Read the model definition and answer for the solid it produces. Units are mm, in the model's axes. Coordinates: 2 decimals unless noted, no trailing zeros.
Q1. Straight lines are drawn through the part: line 1 (Z direction, x = 117, y = -3.75); line 2 (Z direction, x = 168, y = -3.2); line 3 (X direction, y = -2.9, z = -32). For each, find the intervals that lie inside material, in ascending order.
Q2. Section A-A (x = 135.5) is taken. Count the separate pieces of the cut face and the enclosed holes in it, then the cut area to 3 significant figures.
Q3. A flat-ended cylindrical pin translates along its axis: P1, Ø2, axis at y = -1.5, z = -31, coming from the +X side. Find the tip coordinate at first contact, or state that the pin passes through.
from build123d import *

# Parameters (mm, degrees)
F0_R     = 17.789827
F0_R_2   = 16.122829
F0_R_3   = 17.435886
F0_R_4   = 16.480186
F0_R_5   = 13.049133
F1_DEPTH = 4


with BuildPart() as f1:
    # F0 (on Front) → F1 (new body)
    with BuildSketch(Plane.XZ):
        with BuildLine():
            Line((128.107603, -34.568384), (160.109099, -34.568384))
            Line((160.109099, -34.568384), (160.109099, -27.068384))
            Line((160.109099, -27.068384), (174.109099, -27.068384))
            add(Edge.make_bspline(
                [(169.24465, 102.431616), (172.691915, 62.91882), (174.04711, 17.96585), (174.109099, -27.068384)],
                knots=[126.909658, 126.909658, 126.909658, 126.909658, 238.208295, 238.208295, 238.208295, 238.208295], degree=3))
            Line((169.24465, 102.431616), (155.24465, 102.431616))
            Line((155.24465, 102.431616), (155.24465, 109.931616))
            Line((155.24465, 109.931616), (130.150168, 109.931616))
            Line((130.150168, 109.931616), (130.150168, 102.431616))
            Line((130.150168, 102.431616), (116.150168, 102.431616))
            add(Edge.make_bspline(
                [(116.150168, 102.431616), (116.157251, 97.264949), (116.144052, 92.098282), (116.107603, 86.931616)],
                knots=[106.01436, 106.01436, 106.01436, 106.01436, 121.51646, 121.51646, 121.51646, 121.51646], degree=3))
            add(Edge.make_bspline(
                [(116.107603, 86.931616), (115.839525, 48.931616), (114.313799, 10.931616), (114.12646, -27.068384)],
                knots=[121.51646, 121.51646, 121.51646, 121.51646, 235.531904, 235.531904, 235.531904, 235.531904], degree=3))
            Line((114.12646, -27.068384), (128.107603, -27.068384))
            Line((128.107603, -27.068384), (128.107603, -34.568384))
        make_face()
        with Locations((143.329501, 35.698157)):
            Circle(F0_R, mode=Mode.SUBTRACT)
        with Locations((143.329501, 79.504788)):
            Circle(F0_R_2, mode=Mode.SUBTRACT)
        with Locations((144.569308, -4.802315)):
            Circle(F0_R_3, mode=Mode.SUBTRACT)
        with BuildLine():
            Line((155.24465, 117.431616), (167.805281, 117.431616))
            add(Edge.make_bspline(
                [(148.107603, 208.431616), (157.469501, 188.064638), (163.759947, 155.883562), (167.805281, 117.431616)],
                knots=[0, 0, 0, 0, 112.560289, 112.560289, 112.560289, 112.560289], degree=3))
            Line((148.107603, 208.431616), (114.107603, 208.431616))
            add(Edge.make_bspline(
                [(114.107603, 208.431616), (114.96357, 178.098282), (115.819537, 147.764949), (116.075302, 117.431616)],
                knots=[0, 0, 0, 0, 91.012328, 91.012328, 91.012328, 91.012328], degree=3))
            Line((116.075302, 117.431616), (116.150168, 117.431616))
            Line((116.150168, 117.431616), (130.150168, 117.431616))
            Line((130.150168, 117.431616), (130.150168, 109.931616))
            Line((130.150168, 109.931616), (155.24465, 109.931616))
            Line((155.24465, 109.931616), (155.24465, 117.431616))
        make_face()
        with Locations((138.783529, 140.668765)):
            Circle(F0_R_4, mode=Mode.SUBTRACT)
        with Locations((135.477364, 179.929435)):
            Circle(F0_R_5, mode=Mode.SUBTRACT)
        with BuildLine():
            Line((160.109099, -42.068384), (160.109099, -34.568384))
            Line((160.109099, -34.568384), (128.107603, -34.568384))
            Line((128.107603, -34.568384), (128.107603, -42.068384))
            Line((128.107603, -42.068384), (114.12646, -42.068384))
            add(Edge.make_bspline(
                [(114.12646, -42.068384), (114.313799, -80.068384), (115.839525, -118.068384), (116.107603, -156.068384)],
                knots=[250.533936, 250.533936, 250.533936, 250.533936, 364.549379, 364.549379, 364.549379, 364.549379], degree=3))
            add(Edge.make_bspline(
                [(116.107603, -156.068384), (116.144052, -161.235051), (116.157251, -166.401718), (116.150168, -171.568384)],
                knots=[364.549379, 364.549379, 364.549379, 364.549379, 380.051479, 380.051479, 380.051479, 380.051479], degree=3))
            Line((116.150168, -171.568384), (130.150168, -171.568384))
            Line((130.150168, -171.568384), (130.150168, -179.068384))
            Line((130.150168, -179.068384), (130.150168, -186.568384))
            Line((130.150168, -186.568384), (116.150168, -186.568384))
            Line((116.150168, -186.568384), (116.075302, -186.568384))
            add(Edge.make_bspline(
                [(116.075302, -186.568384), (115.819537, -216.901718), (114.96357, -247.235051), (114.107603, -277.568384)],
                knots=[395.053511, 395.053511, 395.053511, 395.053511, 486.065839, 486.065839, 486.065839, 486.065839], degree=3))
            Line((114.107603, -277.568384), (148.107603, -277.568384))
            add(Edge.make_bspline(
                [(167.317003, -186.568384), (163.250156, -224.455468), (157.083255, -256.397009), (148.107603, -277.568384)],
                knots=[377.036866, 377.036866, 377.036866, 377.036866, 488.773976, 488.773976, 488.773976, 488.773976], degree=3))
            Line((167.317003, -186.568384), (155.24465, -186.568384))
            Line((155.24465, -186.568384), (155.24465, -179.068384))
            Line((155.24465, -179.068384), (155.24465, -171.568384))
            Line((155.24465, -171.568384), (168.792157, -171.568384))
            add(Edge.make_bspline(
                [(174.082738, -42.068384), (173.861315, -87.342067), (172.335726, -132.128552), (168.792157, -171.568384)],
                knots=[250.568896, 250.568896, 250.568896, 250.568896, 362.574274, 362.574274, 362.574274, 362.574274], degree=3))
            Line((174.082738, -42.068384), (160.109099, -42.068384))
        make_face()
        with Locations((135.477364, -249.066204)):
            Circle(F0_R_5, mode=Mode.SUBTRACT)
        with Locations((138.783529, -209.805533)):
            Circle(F0_R_4, mode=Mode.SUBTRACT)
        with Locations((143.329501, -148.641557)):
            Circle(F0_R_2, mode=Mode.SUBTRACT)
        with Locations((143.329501, -104.834925)):
            Circle(F0_R, mode=Mode.SUBTRACT)
        with Locations((144.569308, -64.334454)):
            Circle(F0_R_3, mode=Mode.SUBTRACT)
    extrude(amount=F1_DEPTH)


solid = f1.part
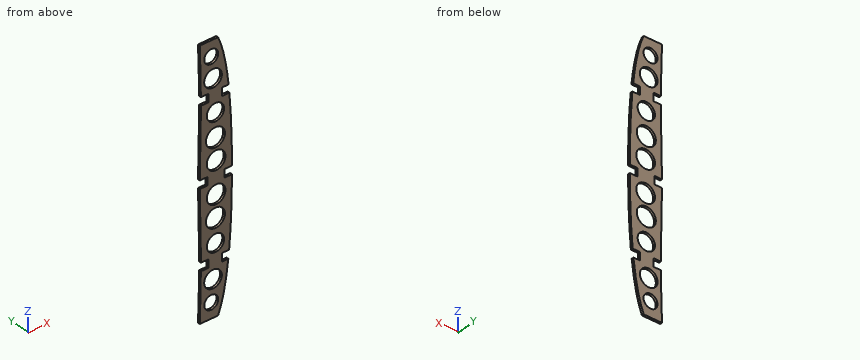
Numbers:
1. line 1: z = -277.57 to -186.57, -171.57 to -42.07, -27.07 to 102.43, 117.43 to 208.43
1. line 2: z = -171.57 to -42.07, -27.07 to 102.43
1. line 3: x = 128.11 to 160.11
2. separate pieces: 11
2. enclosed holes: 0
2. area: 757 mm2
3. P1: stops at x = 160.11
